The model under review builds one solid part; all positions refer to its coordinate system, in mm. A direction names the side the tool comes from. Coordinates: 2 decimals unless noted, no trailing zeros. Loops run counter-clockwise (first coordinate to the right, second up) from the corner with the lowest first, then second, coordinate; pieces in that order, holes last. Notation, with made-up numbers: (13, 41) - (69, 41) arc R13 ccw to (69, 59) - close; hole circle Ø6 at (-9.75, -29.5). An arc over 180 degrees is marked (long way). Answer in a Markdown table with one row per item. Add a question column.
(1) We need section A-A on x = 0. Write out the cut boundary in (y, z).
(2) We need section B-B on y = 0. Write out the cut boundary in (x, z).
(3) For P1, Ø2, axis at x = -8.5, y = 9, coming from the +Z side; P2, Ø4.5, axis at x = 9.19, y = -9.19, coming from the +Z side; P3, Ø12, axis at x = 11, y = 10, coming from the -Z side; P4, Ø4, axis at x = 0.5, y = -10, coming from the +Z side, all flat-tipped, find the tip position at first contact; note any pin that passes through.
(4) Mouldability with a two-part tool opening along X and no side actions: class faces 1 (the cylindrical face through (7.718, 10.544, -2.958)), 2 (the flat face through (-16, 3, -5)), 3 (the cylindrical face through (-3.47, 15.62, -35.53)) as +X half, -X half, draft (parallel to the pull), parting line (faces both ways), or undercut.
(5) We need section C-C on z = -3.5. Write out the cut boundary in (x, y).
(6) We need section D-D on z = -47. Write out the cut boundary in (x, y).
(7) Machinability: for faces 4 (the flat face through (0, -9, 1)), 5 (the cylindrical face through (-1.796, 13.683, -56.734)), 6 (the flat face through (0, 0, 0)), 7 (the cylindrical face through (10, 0, 1)), which of the approach directions +Z, -Z, +X, -X, +Y, -Y give a long, thin tool a straight path to every point of the face, cutting with its end or side? Answer none if there is none.
(8) For line 1 along Z through (x, y) = (1, 15); line 2 along Z through (x, y) = (8.5, 9.5); line 3 along Y through (x, z) = (-9.5, -27.5), list the stretches that pass through material, from the lowest coordinate up.
Autodesk Inventor part; units mm, degrees
ref_plane "Work Plane1" through (0, 0, -38) normal (0, 0, 1) x (1, 0, 0)
ref_plane "Work Plane2" through (0, 0, -5) normal (0, 0, 1) x (1, 0, 0)
ref_plane "Work Plane3" through (0, 0, -33) normal (0, 0, -1) x (-1, 0, 0)
sketch "Sketch1" plane through (0, 0, 0) normal (0, 0, 1) x (1, 0, 0)
  circle A0 centre (0, 0) radius 13.8
  dimension "d0" = 27.6
extrude "Extrusion1" add sketch "Sketch1" against normal blind 76
ref_plane "Work Plane1" through (0, 0, -38) normal (0, 0, 1) x (1, 0, 0)
sketch "Sketch2" plane through (0, 0, -38) normal (0, 0, 1) x (1, 0, 0)
  circle A0 centre (0, 0) radius 13.8
  circle A1 centre (0, 0) radius 16
  dimension "d4" = 32
extrude "Extrusion2" add sketch "Sketch2" along normal blind 38
sketch "Sketch3" plane through (0, 0, -76) normal (0, 0, -1) x (-1, 0, 0)
  circle A0 centre (0, 0) radius 5
  dimension "d7" = 10
extrude "Extrusion3" add sketch "Sketch3" along normal blind 2
sketch "Sketch4" plane through (0, 0, 0) normal (0, 0, 1) x (1, 0, 0)
  circle A0 centre (0, 0) radius 5
  circle A1 centre (0, 0) radius 10
  line L0 (-4.3589, -9) -> (4.3589, -9)
  line L1 (4.3589, -9) -> (4.3589, 9)
  line L2 (4.3589, 9) -> (-4.3589, 9)
  line L3 (-4.3589, 9) -> (-4.3589, -9)
  line L4 (-4.3589, -9) -> (4.3589, 9) construction
  line L5 (4.3589, -9) -> (-4.3589, 9) construction
  dimension "d10" = 20
  dimension "d11" = 18
extrude "Extrusion4" add sketch "Sketch4" along normal blind 3 contours A0 L1 | A0 L1 A1 | L1 A0 L3 | A0 L3 L2 L1 | L1 L0 L3 A0 | L3 A0 | A0 L3 A1
sketch "Sketch5" plane through (0, 0, 3) normal (0, 0, 1) x (1, 0, 0)
  circle A0 centre (0, 0) radius 3
  dimension "d14" = 6
extrude "Extrusion5" cut sketch "Sketch5" against normal blind 3
sketch "Sketch6" plane through (0, 0, 0) normal (0, 0, 1) x (1, 0, 0)
  circle A0 centre (0, 0) radius 3
  circle A1 centre (0, 0) radius 13
  line L0 (0, 0) -> (9.1924, 9.1924)
  line L1 (0, 0) -> (13, 0) construction
  circle A2 centre (9.1924, 9.1924) radius 2
  dimension "d17" = 26
  dimension "d18" = 45
  dimension "d19" = 4
extrude "Extrusion6" cut sketch "Sketch6" against normal blind 6 contours A2 A1 L0 | L0 A1 A2 | A1 A2 picked at (9.9348, 9.3429)
pattern_circular "Circular Pattern1" count 4 over 360 about axis through (0, 0, -38) along (0, 0, 1) of "Extrusion6"
ref_plane "Work Plane2" through (0, 0, -5) normal (0, 0, 1) x (1, 0, 0)
ref_plane "Work Plane3" through (0, 0, -33) normal (0, 0, -1) x (-1, 0, 0)
sketch "Sketch7" plane through (0, 0, -5) normal (0, 0, 1) x (1, 0, 0)
  circle A0 centre (9.1924, -9.1924) radius 2
  circle A1 centre (-9.1924, -9.1924) radius 2
  circle A2 centre (-9.1924, 9.1924) radius 2
  circle A3 centre (9.1924, 9.1924) radius 2
  line L0 (4.3589, -9) -> (-4.3589, -9)
  arc A4 (-4.3589, 9) -> (-4.3589, -9) centre (0, 0) ccw
  line L1 (-4.3589, 9) -> (4.3589, 9)
  arc A5 (4.3589, -9) -> (4.3589, 9) centre (0, 0) ccw
  circle A6 centre (0, 0) radius 16
  circle A7 centre (0, 0) radius 3
  circle A8 centre (0, 0) radius 16.5
  dimension "d27" = 33
extrude "Extrusion7" add sketch "Sketch7" against normal up to surface (28 mm away) contours A8
thread "Thread1"
thread "Thread2"
thread "Thread3"
thread "Thread4"
properties part number "motor_body" material "Steel, Mild"
Outcome:
| question | item | result |
|---|---|---|
| 1 | outline | (-16.5, -33) - (-16, -33) - (-16, -38) - (-13.8, -38) - (-13.8, -76) - (-5, -76) - (-5, -78) - (5, -78) - (5, -76) - (13.8, -76) - (13.8, -38) - (16, -38) - (16, -33) - (16.5, -33) - (16.5, -5) - (16, -5) - (16, 0) - (9, 0) - (9, 3) - (3, 3) - (3, 0) - (-3, 0) - (-3, 3) - (-9, 3) - (-9, 0) - (-16, 0) - (-16, -5) - (-16.5, -5) - close |
| 2 | outline | (-16.5, -33) - (-16, -33) - (-16, -38) - (-13.8, -38) - (-13.8, -76) - (-5, -76) - (-5, -78) - (5, -78) - (5, -76) - (13.8, -76) - (13.8, -38) - (16, -38) - (16, -33) - (16.5, -33) - (16.5, -5) - (16, -5) - (16, 0) - (10, 0) - (10, 3) - (3, 3) - (3, 0) - (-3, 0) - (-3, 3) - (-10, 3) - (-10, 0) - (-16, 0) - (-16, -5) - (-16.5, -5) - close |
| 3 | P1 | z = -6 |
| 3 | P2 | z = 0 |
| 3 | P3 | z = -76 |
| 3 | P4 | z = 3 |
| 4 | face 1 | undercut |
| 4 | face 2 | draft |
| 4 | face 3 | parting line |
| 5 | outline | circle Ø32 at (0, 0); hole circle Ø4 at (-9.19, -9.19); hole circle Ø4 at (-9.19, 9.19); hole circle Ø4 at (9.19, -9.19); hole circle Ø4 at (9.19, 9.19) |
| 6 | outline | circle Ø27.6 at (0, 0) |
| 7 | face 4 | +Z, +X, -X, -Y |
| 7 | face 5 | -Z |
| 7 | face 6 | +Z |
| 7 | face 7 | +Z, +X |
| 8 | line 1 | -38 to 0 |
| 8 | line 2 | -76 to -6 |
| 8 | line 3 | -13.49 to 13.49 |
